from build123d import *

# Parameters (mm, degrees)
SKETCH1_W           = 22
SKETCH1_H           = 18
SKETCH1_R           = 2
BOSS_EXTRUDE2_DEPTH = 3
SKETCH2_W           = 2
SKETCH2_H           = 18
BOSS_EXTRUDE3_DEPTH = 24
SKETCH3_R           = 2.5
CUT_EXTRUDE1_DEPTH  = 24


with BuildPart() as part:
    # Sketch1 → Boss-Extrude2 (new body)
    with BuildSketch(Plane(origin=(0, 0, 0), x_dir=(1, 0, 0), z_dir=(0, 1, 0))):
        Rectangle(SKETCH1_W, SKETCH1_H)
        with Locations(Location((0, 0, 0), (0, 0, 270))):
            Circle(SKETCH1_R, mode=Mode.SUBTRACT)
    boss_extrude2 = extrude(amount=BOSS_EXTRUDE2_DEPTH)

    # Sketch2 → Boss-Extrude3 (add)
    with BuildSketch(Plane(origin=(0, 3, 0), x_dir=(1, 0, 0), z_dir=(0, 1, 0))):
        with Locations((-10, 0)):
            Rectangle(SKETCH2_W, SKETCH2_H)
    boss_extrude3 = extrude(amount=BOSS_EXTRUDE3_DEPTH)

    # Sketch3 → Cut-Extrude1 (cut)
    with BuildSketch(Plane.ZY.offset(11)):
        with BuildLine():
            Line((9, 27), (0, 27))
            ThreePointArc((0, 27), (6.363961031, 24.363961031), (9, 18))
            Line((9, 18), (9, 27))
        make_face()
        with BuildLine():
            Line((-9, 27), (-9, 18))
            ThreePointArc((-9, 18), (-6.363961031, 24.363961031), (0, 27))
            Line((0, 27), (-9, 27))
        make_face()
        with Locations((0, 18)):
            Circle(SKETCH3_R)
    cut_extrude1 = extrude(amount=-CUT_EXTRUDE1_DEPTH, mode=Mode.SUBTRACT)

    # Mirror1: Boss-Extrude2, Boss-Extrude3, Cut-Extrude1 across plane
    add(boss_extrude2.mirror(Plane(origin=(0, 0, 0), x_dir=(0, 0, 1), z_dir=(1, 0, 0))))
    add(boss_extrude3.mirror(Plane(origin=(0, 0, 0), x_dir=(0, 0, 1), z_dir=(1, 0, 0))))
    add(cut_extrude1.mirror(Plane(origin=(0, 0, 0), x_dir=(0, 0, 1), z_dir=(1, 0, 0))), mode=Mode.SUBTRACT)


solid = part.part
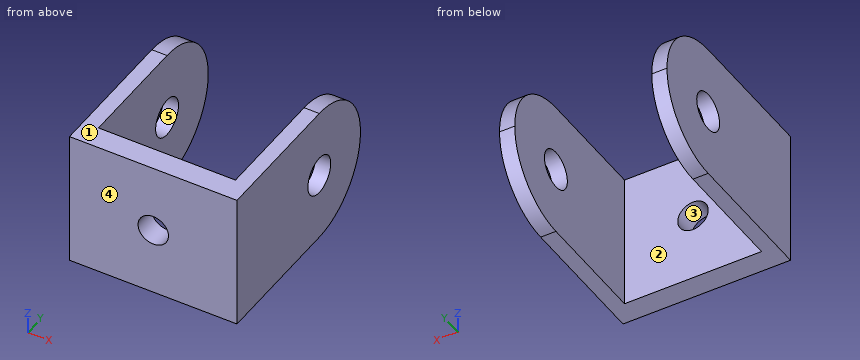
Design review of the part built by this model. Coordinates are the model's own, in mm. Face numbers are marked on the shaded views. A direction names the side the tool comes from. Round coordinates to 2 decimals unless told otherwise and drop trailing zeros. Write each loop counter-clockwise with the first axis right and the second up, starting at its lowest first coordinate (ties: lowest second). Pieces come first, ordered by that corner, then holes. Notation, with made-up numbers: M -31.75,67 L 24.25,67 A10 ccw 24.25,84 Z; hole C 0.5,57 d1. An arc over 180 degrees is marked long. One line per item, written item: value. Start each with the question number.
1. Take a section at D-D on z = 7.75. State the section outline as (x, y) points, then the cut area to 3 significant figures.
2. For the marked faces 1 and 2, list the 3-axis set-ups (+Z, -Z, +X, -X, +Y, -Y) from which the entire face can be reached by the end or side of a thin tool; tool diameter is ignored.
3. To check wall thickness, follow probe 1 along X at (y, z) = (4.5, -3.75); probe 2 along Z at (x, y) = (10.1, 18); probe 3 along Y at (x, z) = (4.25, -2.75). State the ranges of each line that lie inside material, in increasing order. Write a range as from..to.
4. Draft analysis for pull direction Y (two halves, no side actions). For the marked faces 3, 4 and 5, state which applies: pulls with the +Y half, pulls with the -Y half, needs draft (parallel to the pull), parting line crosses it, or undercut.
5. Clearance check with flat-ended pins moving along their axes: P1, Ø8, axis at y = 18, z = 0, coming from the -X side; P2, Ø1.5, axis at x = 6, z = 6, coming from the +Y side. State where each tip first meets the part, or that it passes through.
6. Take a section at B-B on y = 11.75. State the section outline as (x, z) points, then the cut area to 3 significant figures.
7. Take a section at A-A on x = 0. State the section outline as (y, z) points.
8. Take a section at C-C on z = 1. State the section outline as (x, y) points.
Computed:
1. outline: M -11,0 L 11,0 L 11,22.58 L 9,22.58 L 9,3 L -9,3 L -9,22.58 L -11,22.58 Z
1. area: 144 mm²
2. face 1: +Z, +X, -X, +Y, -Y
2. face 2: +Z, -Z, +Y
3. probe 1: x = -11..-9, 9..11
3. probe 2: z = -9..-2.5, 2.5..9
3. probe 3: y = 0..3
4. face 3: needs draft
4. face 4: pulls with the -Y half
4. face 5: undercut
5. P1: stops at x = -11
5. P2: stops at y = 3
6. outline: M -11,-9 L -9,-9 L -9,9 L -11,9 Z; M 9,-9 L 11,-9 L 11,9 L 9,9 Z
6. area: 72.0 mm²
7. outline: M 0,-9 L 3,-9 L 3,-2 L 0,-2 Z; M 0,2 L 3,2 L 3,9 L 0,9 Z
8. outline: M -11,0 L -1.73,0 L -1.73,3 L -9,3 L -9,15.71 L -11,15.71 Z; M -11,20.29 L -9,20.29 L -9,26.94 L -11,26.94 Z; M 1.73,0 L 11,0 L 11,15.71 L 9,15.71 L 9,3 L 1.73,3 Z; M 9,20.29 L 11,20.29 L 11,26.94 L 9,26.94 Z
